```python
from build123d import *

# Parameters (mm, degrees)
F1_DEPTH        = 63.5
F0_W            = 25.4
F0_H            = 19.0499989867
F2_DEPTH        = 25.4
F3_DEPTH        = 7.9375
F6_D            = 6.35
F6_CSINK_D      = 12.7
F6_CSINK_ANGLE  = 90
F7_COUNT        = 3
F9_D            = 6.35
F9_COPIES_COUNT = 3
F10_R           = 25.4


# Not quite as in the source:
# - a pattern or mirror of a feature is missing from the dataset's text; its kind, count and spacing are read off the source's solid


with BuildPart() as f1:
    # F0 (on Front) → F1 (new body, symmetric)
    with BuildSketch(Plane.XZ):
        Polygon((50.8, -12.7), (50.8, 12.7), (31.7500010133, 12.7), (-50.8, 12.7), (-50.8, -12.7), align=None)
    extrude(amount=F1_DEPTH, both=True)

    # F0 (on Front) → F2 (join, symmetric)
    with BuildSketch(Plane.XZ):
        with BuildLine():
            Line((31.7500010133, 12.7), (50.8, 12.7))
            Line((50.8, 12.7), (50.8, 38.1))
            ThreePointArc((50.8, 38.1), (54.5197438789, 47.0802561211), (63.5, 50.8))
            Line((63.5, 50.8), (76.2, 50.8))
            Line((76.2, 50.8), (76.2, 69.8499989867))
            Line((76.2, 69.8499989867), (63.5, 69.8499989867))
            add(Edge.make_bspline(
                [(60.7424728123, 69.7300249678), (61.6706362679, 69.7791364012), (62.5900608791, 69.8191720775), (63.5, 69.8499989867)],
                knots=[125.2378350903, 125.2378350903, 125.2378350903, 125.2378350903, 127.791284461, 127.791284461, 127.791284461, 127.791284461], degree=3))
            ThreePointArc((60.7424728123, 69.7300249678), (40.0947236603, 59.5535655573), (31.7500010133, 38.1))
            Line((31.7500010133, 38.1), (31.7500010133, 12.7))
        make_face()
        with Locations((88.9, 60.3249994934)):
            Rectangle(F0_W, F0_H)
    extrude(amount=F2_DEPTH, both=True)

    # F0 (on Front) → F3 (join, symmetric)
    with BuildSketch(Plane.XZ):
        with BuildLine():
            Line((-50.8, 12.7), (31.7500010133, 12.7))
            Line((31.7500010133, 12.7), (31.7500010133, 38.1))
            ThreePointArc((31.7500010133, 38.1), (40.0947236603, 59.5535655573), (60.7424728123, 69.7300249678))
            add(Edge.make_bspline(
                [(-50.8, 12.7), (-51.3257578554, 43.0802353164), (15.219274615, 67.3212795022), (60.7424728123, 69.7300249678)],
                knots=[0, 0, 0, 0, 125.2378350903, 125.2378350903, 125.2378350903, 125.2378350903], degree=3))
        make_face()
    extrude(amount=F3_DEPTH, both=True)

    # F0 (on Front) → F4 (revolve)
    with BuildSketch(Plane.XZ):
        Polygon((101.6, 69.8499989867), (101.6, 50.8), (101.6, 44.45), (127, 44.45), (127, 76.2), (101.6, 76.2), align=None)
    revolve(axis=Axis((101.6, 0, 60.325), (0, 0, -1)))

    # F6 (through all)
    with Locations(Plane.XY.offset(12.7)):
        with Locations((-27.541898191, -35.71875), (-27.541898191, 38.6316925287)):
            CounterSinkHole(F6_D / 2, F6_CSINK_D / 2, counter_sink_angle=F6_CSINK_ANGLE)

    # F7: F1 ×3 about axis
    f7_axis = Axis((101.6, 0, 60.325), (0, 0, -1))


with BuildPart() as f1_1:
    add(f1.part)
    for i in range(1, F7_COUNT):
        add(f1.part.rotate(f7_axis, i * 360 / F7_COUNT))

    # F9 (through all)
    with Locations(Plane.XY.offset(76.2)):
        with Locations((81.3262090087, 0)):
            f9 = Hole(F9_D / 2)

    # F9_copies: F9 ×3 about axis
    f9_copies_axis = Axis((101.6, 0, 0), (0, 0, 1))
    for i in range(1, F9_COPIES_COUNT):
        add(f9.rotate(f9_copies_axis, i * 360 / F9_COPIES_COUNT), mode=Mode.SUBTRACT)

    # F10
    f10_edges = [f1_1.edges().sort_by_distance(p)[0] for p in [
        (-50.8, -63.5, 0),
        (122.807387, -163.732272, 0),
        (232.792613, -100.232272, 0),
        (232.792613, 100.232272, 0),
        (181.992613, 12.244091, 0),
        (181.992613, -12.244091, 0),
        (50.8, -63.5, 0),
        (122.807387, 163.732272, 0),
        (72.007387, 75.744091, 0),
        (72.007387, -75.744091, 0),
        (50.8, 63.5, 0),
        (-50.8, 63.5, 0),
    ]]
    fillet(f10_edges, radius=F10_R)


solid = f1_1.part
```
The model under review builds one solid part; all positions refer to its coordinate system, in mm. A direction names the side the tool comes from. Give positions to 0.01 mm unless a question says otherwise; leave off trailing zeros. Write each question's results on one line, items separated by ' | '. Start each with the question number.
1. Insertion check: pin 1 Ø4 at (x, z) = (47, 42) entering from +Y; pin 2 Ø1.5 at (x, z) = (105, -1) entering from +Y; pin 3 Ø10 at (x, y) = (81.33, 0) entering from +Z; pin 4 Ø1 at (x, y) = (168.5, 20) entering from -Z. Each pin has a flat end and moves straight along its axis. Give the tip position at first contact, or say it passes through.
2. For probe 1 along Y at (x, z) = (-29, -5); probe 2 along X at (y, z) = (-4.5, 8); probe 3 along Z at (x, y) = (89, 87.5), list the stretches that pass through material, from the lowest coordinate up. Write a range as [from, to].
3. We need section A-A (z = -1.5). Count the separate pieces of the cut face and the enclosed holes in it, and give its area (3 significant figures).
4. Mouldability with a two-part tool opening along Y and no side actions: class faces 6 (the cylindrical face through (125.063, 9.728, 73.069)), 7 (the flat face through (121.98, 68.89, 25.58)), 8 (the cylindrical face through (125.5, -40.68, 46.98)) as released by +Y, released by -Y, zero draft, split by the parting line, or undercut.
5. For faces 1 (the cylindrical face through (117.699, 61.467, 59.796)), 2 (the flat face through (143.564, -88.559, 35.278)), 3 (the flat face through (4, 7.938, 35)), 4 (the flat face through (183, 70, 12.7)), 5 (the cylindrical face through (43.56, -55.86, 0.18)), list the 3-axis set-ups (+Z, -Z, +X, -X, +Y, -Y) from which the entire face can be reached by the end or side of a thin tool; tool diameter is ignored.
Results found:
1) pin 1: stops at y = 25.4 | pin 2: stops at y = 134.19 | pin 3: stops at z = 76.2 | pin 4: passes through
2) probe 1: y = [-63.24, -38.54], [-32.9, 35.81], [41.45, 63.24] | probe 2: x = [-50.8, 50.8] | probe 3: z = [-12.7, 12.7]
3) separate pieces: 3 | enclosed holes: 6 | area: 36,900 mm^2
4) face 6: split by the parting line | face 7: released by +Y | face 8: undercut
5) face 1: +Z, +Y | face 2: +Z, -Y | face 3: +Z, -X, +Y | face 4: +Z, +X | face 5: +Z, -Z, -Y
